Read the model definition and answer for the solid it produces. Units are mm, in the model's axes. A direction names the side the tool comes from. Coordinates: 2 decimals unless noted, no trailing zeros. Order: outer loops, then holes, each group sorted by start corner. A loop starts at its lowest first (then second) coordinate and runs counter-clockwise, first axis right, second up. Notation, with made-up numbers: M 10.5,-15.5 L 36.5,-15.5 A25 cw 36.5,21.5 Z; hole C 69,-35 d11. An arc over 180 degrees is marked long. One line per question, with ' | ' between items. Start each with the question number.
1) A tool of negligible diameter and unlimited length cuts with its end or side. For faces 1 (the face through (2.6, 0.6, 4.7)), 2 (the face through (2.7, 0, 4.7)), 3 (the face through (2.6, 10, 4.7)), 4 (the face through (-0.015, 0.304, 4.699)), 5 (the face through (0, 5, 0)), from which of +Z, -Z, +X, -X, +Y, -Y can it reach the whole face along a straight path? Write none if from no direction.
2) Find section A-A, the plane x = 3.5. Write down the section's boundary in (y, z).
3) Find section C-C, the plane z = 2.1. Write down the section's boundary in (x, y), plus the area to 3 significant figures.
4) Find section B-B, the plane x = 0. Write down the section's boundary in (y, z), plus the area to 3 significant figures.
5) Given P1, Ø0.5, axis at x = 2.5, y = 3.5, coming from the -Z side; P2, Ø0.7, axis at y = 9.5, z = 3.5, coming from the +X side; P3, Ø1, axis at x = 2.5, z = 4, coming from the -Y side, each flat-ended and moving along its own axis, determine where each tip first touches the part or whether it passes through.
6) Find section D-D, the plane y = 5.5. Write down the section's boundary in (x, z).
7) Consider probe 1 along Y at (x, z) = (5.75, 4.6); probe 2 along X at (y, z) = (6.75, 2.35); probe 3 along Z at (x, y) = (4.75, 3.25). Determine where each line is inside the solid, lowest interval first.
Autodesk Inventor part; units mm, degrees
ref_plane "YZ Plane" through (0, 0, 0) normal (1, 0, 0) x (0, 1, 0)
ref_plane "XZ Plane" through (0, 0, 0) normal (0, 1, 0) x (-1, 0, 0)
ref_plane "XY Plane" through (0, 0, 0) normal (0, 0, 1) x (1, 0, 0)
sketch "Esboço1" plane through (0, 0, 0) normal (0, 0, 1) x (1, 0, 0)
  line L0 (0, 0) -> (0, 10) construction
  line L1 (1, 0) -> (1, 10)
  line L2 (-1, 10) -> (-1, 0)
  arc A0 (-1, 0) -> (1, 0) centre (0, 0) ccw
  arc A1 (1, 10) -> (-1, 10) centre (0, 10) ccw
  point P0 (0, 5)
  dimension "d0" = 10
  dimension "d1" = 2
extrude "Extrusão1" add sketch "Esboço1" along normal blind 3
sketch "Esboço2" plane through (0, 0, 3) normal (0, 0, 1) x (1, 0, 0)
  arc A0 (1, 10) -> (-1, 10) centre (0, 10) ccw construction
  arc A1 (-1, 0) -> (1, 0) centre (0, 0) ccw construction
  line L0 (0, 10) -> (0, 0) construction
  line L1 (-1, 10) -> (-1, 0) construction
  line L2 (-1, 0) -> (1, 0) construction
  line L3 (0.3, 0) -> (-0.3, 0)
  line L4 (-0.3, 0) -> (-0.3, 0.6)
  line L5 (-0.3, 0.6) -> (0.3, 0.6)
  line L6 (0.3, 0.6) -> (0.3, 0)
  dimension "d4" = 0.6
  dimension "d5" = 0.6
  dimension "d6" = 0.6
  dimension "d7" = 0.3
extrude "Extrusão2" add sketch "Esboço2" along normal blind 2
sketch "Esboço3" plane through (0, 0, 5) normal (0, 0, 1) x (1, 0, 0)
  line L0 (0.3, 0) -> (-0.3, 0)
  line L1 (-0.3, 0.6) -> (0.3, 0.6)
  line L2 (0.3, 0.6) -> (0.3, 0)
  line L3 (0.3, 0.6) -> (0.3, 0)
  line L4 (0.3, 0.6) -> (7.3, 0.6)
  line L5 (7.3, 0.6) -> (7.3, 0)
  line L6 (7.3, 0) -> (0.3, 0)
  line L7 (0.3, 0) -> (0.3, 0.6)
  point P0 (0, 0)
  dimension "d13" = 7
extrude "Extrusão3" add sketch "Esboço3" against normal blind 0.6
fillet "Arredondamento1" radius 1 1 edges at (-0.3, 0.3, 5)
pattern_linear "Padrão retangular1" count 4 spacing 3.1333 along (0, 1, 0) of "Extrusão3", "Arredondamento1", "Extrusão2"
properties part number "Conector"
Report:
1) face 1: +Z, +X, -X | face 2: +Z, +X, -X, -Y | face 3: +Z, +X, -X, +Y | face 4: +Z, -X, +Y, -Y | face 5: -Z, +X, -X, +Y, -Y
2) outline: M 0,4.4 L 0.6,4.4 L 0.6,5 L 0,5 Z; M 3.13,4.4 L 3.73,4.4 L 3.73,5 L 3.13,5 Z; M 6.27,4.4 L 6.87,4.4 L 6.87,5 L 6.27,5 Z; M 9.4,4.4 L 10,4.4 L 10,5 L 9.4,5 Z
3) outline: M -1,0 A1 ccw 1,0 L 1,10 A1 ccw -1,10 Z | area: 23.1 mm^2
4) outline: M -1,0 L 11,0 L 11,3 L 10,3 L 10,4.71 L 9.4,4.71 L 9.4,3 L 6.87,3 L 6.87,4.71 L 6.27,4.71 L 6.27,3 L 3.73,3 L 3.73,4.71 L 3.13,4.71 L 3.13,3 L 0.6,3 L 0.6,4.71 L 0,4.71 L 0,3 L -1,3 Z | area: 40.1 mm^2
5) P1: stops at z = 4.4 | P2: stops at x = 0.3 | P3: stops at y = 0
6) outline: M -1,0 L 1,0 L 1,3 L -1,3 Z
7) probe 1: y = 0 to 0.6, 3.13 to 3.73, 6.27 to 6.87, 9.4 to 10 | probe 2: x = -1 to 1 | probe 3: z = 4.4 to 5
